Verification items for this drawing (mm, ordinates from the low corner). Round coordinates to 2 decimals unless told otherwise and drop trailing zeros. Order: outer loops, then holes, each group sorted by start corner. A loop starts at its lowest first (then second) coordinate and runs counter-clockwise, first axis right, second up. Notation, with made-up numbers: (-20.5, 7.5) -> (8.5, 7.5) arc R14 cw to (8.5, 12.5) -> close; hole circle Ø8 at (-28, -19). An arc over 180 degrees is marked (long way). Answer in a Markdown table with one row per item. Add a question column.
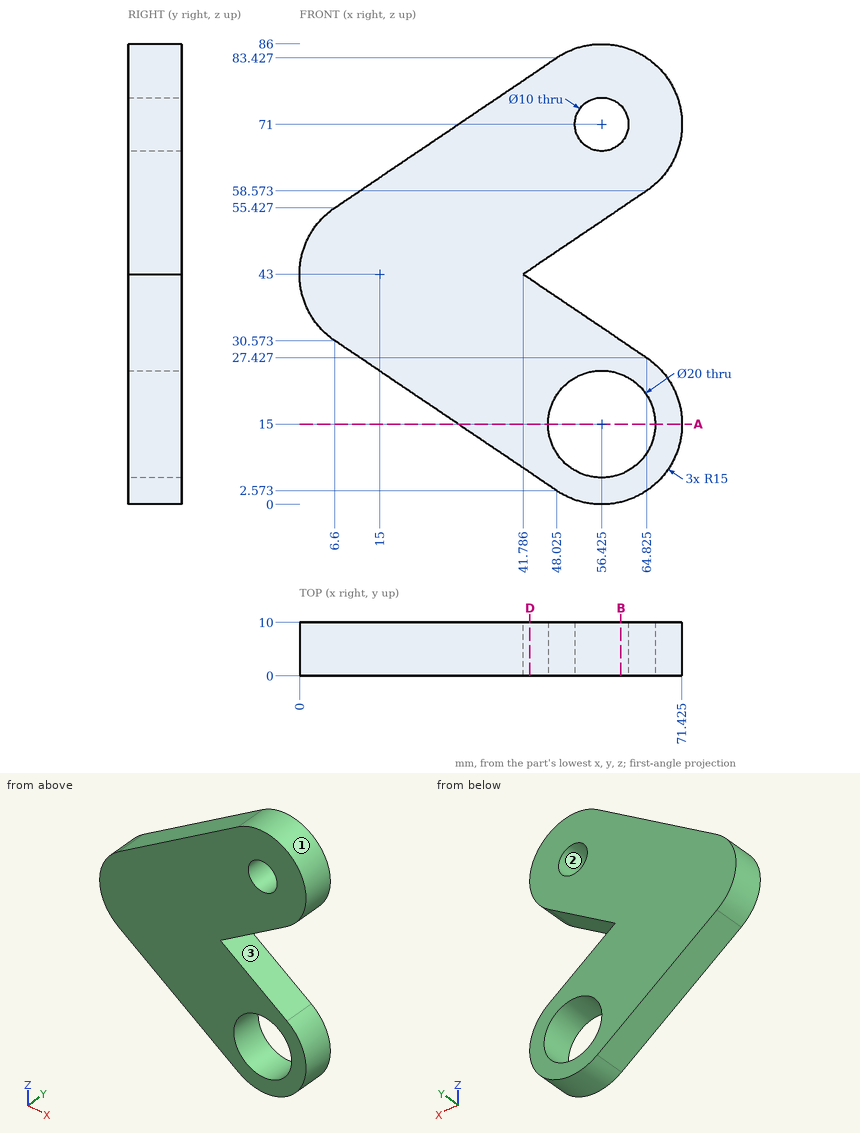
1) Cross-section at D-D, the plane x = 43. Record the boundary of the cut face in (y, z), and give its area (3 significant figures).
2) Cross-section at B-B, the plane x = 60. Record the boundary of the cut face in (y, z) (1 decimal).
3) Cross-section at A-A, the plane z = 15. Record the boundary of the cut face in (x, y) (1 decimal).
4) Depth check by flat-ended pin: P1, Ø1, axis at y = 8, z = 36.5, coming from the +X side; P2, Ø2, axis at y = 2, z = 39.5, coming from the -X side; P3, Ø4, axis at y = 7.5, z = 58, coming from the -X side. Enter the tip coordinate at first touch or a pass-through.
5) Thickness scan on L1, parallel to Z at x = 63.5, y = 9.25 (1 decimal); L2, parallel to X at y = 2.5, z = 15 (1 decimal); L3, parallel to Z at x = 51, y = 5 (1 decimal). Record the ranges inside material, lowest first. Write a range as [from, to].
6) Draft check along X on the marked faces 1, 2 and 3. Enter one of: +X half, -X half, draft (parallel to the pull), parting line (faces both ways), or undercut.
Results below:
| question | item | result |
|---|---|---|
| 1 | outline | (0, 5.97) -> (10, 5.97) -> (10, 42.18) -> (0, 42.18) -> close; (0, 43.82) -> (10, 43.82) -> (10, 80.03) -> (0, 80.03) -> close |
| 1 | area | 724 mm² |
| 2 | outline | (0, 0.4) -> (10, 0.4) -> (10, 5.7) -> (0, 5.7) -> close; (0, 24.3) -> (10, 24.3) -> (10, 30.7) -> (0, 30.7) -> close; (0, 55.3) -> (10, 55.3) -> (10, 67.5) -> (0, 67.5) -> close; (0, 74.5) -> (10, 74.5) -> (10, 85.6) -> (0, 85.6) -> close |
| 3 | outline | (29.6, 0) -> (46.4, 0) -> (46.4, 10) -> (29.6, 10) -> close; (66.4, 0) -> (71.4, 0) -> (71.4, 10) -> (66.4, 10) -> close |
| 4 | P1 | x = 52.14 |
| 4 | P2 | x = 0.21 |
| 4 | P3 | x = 7.45 |
| 5 | L1 | [1.8, 7.9], [22.1, 28.3], [57.7, 84.2] |
| 5 | L2 | [29.6, 46.4], [66.4, 71.4] |
| 5 | L3 | [1, 6.6], [23.4, 36.8], [49.2, 85] |
| 6 | face 1 | parting line |
| 6 | face 2 | undercut |
| 6 | face 3 | +X half |
